For this review, take the finished solid that the model builds, in its own axes (mm). Face numbers are marked on the shaded views. A direction names the side the tool comes from. Round coordinates to 2 decimals unless told otherwise and drop trailing zeros. Order: outer loops, then holes, each group sorted by start corner. A loop starts at its lowest first (then second) coordinate and runs counter-clockwise, first axis right, second up. Notation, with made-up numbers: M -28.5,-6 L -17.5,-6 A22 cw -17.5,4 Z; hole C 48,75 d2. An arc over 180 degrees is marked long. Use a Markdown table: item, result.
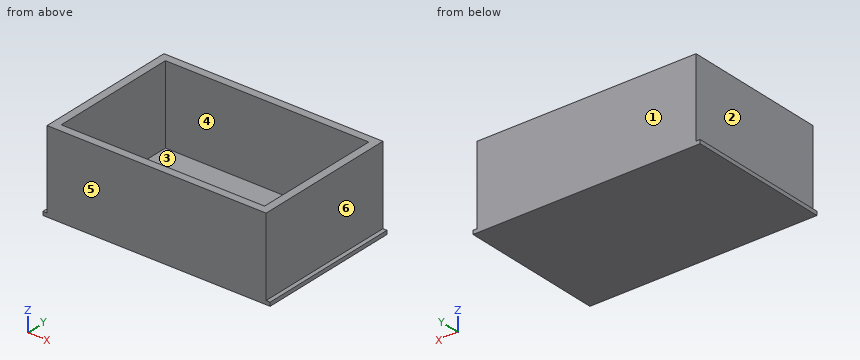
from build123d import *

# Parameters (mm, degrees)
F0_W     = 368.3
F0_H     = 234.95
F1_DEPTH = 6.096
F2_W     = 12.7
F2_H     = 209.55
F3_DEPTH = 127


with BuildPart() as f1:
    # F0 (on Top) → F1 (new body)
    with BuildSketch(Plane.XY):
        Rectangle(F0_W, F0_H)
    extrude(amount=F1_DEPTH)

    # F2 (on face) → F3 (join)
    with BuildSketch(Plane.XY.offset(6.096)):
        with Locations((171.196, 0)):
            Rectangle(F2_W, F2_H)
        Polygon((177.546, 104.775), (177.546, 117.475), (-177.546, 117.475), (-177.546, 104.775), (-164.846, 104.775), (164.846, 104.775), align=None)
        with Locations((-171.196, 0)):
            Rectangle(F2_W, F2_H)
        Polygon((177.546, -117.475), (177.546, -104.775), (164.846, -104.775), (-164.846, -104.775), (-177.546, -104.775), (-177.546, -117.475), align=None)
    extrude(amount=F3_DEPTH)


solid = f1.part
Q1. Draft analysis for pull direction X (two halves, no side actions). For the marked faces 1, 2 and 3, state which applies: pulls with the +X half, pulls with the -X half, needs draft (parallel to the pull), parting line crosses it, or undercut.
Determined:
| item | result |
|---|---|
| face 1 | needs draft |
| face 2 | pulls with the -X half |
| face 3 | undercut |
Q2. Machinability: for the marked faces 4, 5 and 6, which of the approach directions +Z, -Z, +X, -X, +Y, -Y give a long, thin tool a straight path to every point of the face, cutting with its end or side? Answer none if there is none.
Determined:
| item | result |
|---|---|
| face 4 | +Z |
| face 5 | +Z, -Z, +X, -X, -Y |
| face 6 | +Z, +X, +Y, -Y |
Q3. Wall thickness on line 1 along Y through (x, z) = (91.5, 71) (3 decimals); line 2 along X through (y, z) = (5, 27); line 3 along Z through (x, y) = (54.5, 58): over which ranges is each line inside the solid? List them lowest first. Write a range as [from, to].
Determined:
| item | result |
|---|---|
| line 1 | y = [-117.475, -104.775], [104.775, 117.475] |
| line 2 | x = [-177.55, -164.85], [164.85, 177.55] |
| line 3 | z = [0, 6.1] |
Q4. Add section B-B (x = -136). Write out the cut boundary in (y, z) (3 decimals), then the cut area to 3 significant figures.
Determined:
| item | result |
|---|---|
| outline | M -117.475,0 L 117.475,0 L 117.475,133.096 L 104.775,133.096 L 104.775,6.096 L -104.775,6.096 L -104.775,133.096 L -117.475,133.096 Z |
| area | 4,660 mm^2 |
Q5. Add section C-C (y = -19). Write out the cut boundary in (x, z), then the cut area to 3 significant figures.
Determined:
| item | result |
|---|---|
| outline | M -184.15,0 L 184.15,0 L 184.15,6.1 L 177.55,6.1 L 177.55,133.1 L 164.85,133.1 L 164.85,6.1 L -164.85,6.1 L -164.85,133.1 L -177.55,133.1 L -177.55,6.1 L -184.15,6.1 Z |
| area | 5,470 mm^2 |
Q6. Add section A-A (z = 62.5). Write out the cut boundary in (x, y) (3 decimals).
Determined:
| item | result |
|---|---|
| outline | M -177.546,-117.475 L 177.546,-117.475 L 177.546,117.475 L -177.546,117.475 Z; hole M -164.846,-104.775 L 164.846,-104.775 L 164.846,104.775 L -164.846,104.775 Z |
Q7. Clearance check with flat-ended pins moving along their axes: pin 1 (6 mm diameter, centred on x = 100, y = 90, fed in from +Z); pin 2 (1 mm diameter, centred on y = 71.5, z = 113, fed in from +X); pin 3 (1 mm diameter, centred on y = 69.5, z = 83.5, fed in from -X). State where each tip first meets the part, or that it passes through.
Determined:
| item | result |
|---|---|
| pin 1 | stops at z = 6.1 |
| pin 2 | stops at x = 177.55 |
| pin 3 | stops at x = -177.55 |
